Build history of the part. All positions in model axes, mm. Round coordinates to 2 decimals unless told otherwise and drop trailing zeros. Order: outer loops, then holes, each group sorted by start corner. A loop starts at its lowest first (then second) coordinate and runs counter-clockwise, first axis right, second up. Notation, with made-up numbers: (-3.5, -26) -> (54.5, -26) arc R20 ccw to (54.5, -8) -> close; hole circle Ø1 at (84, 65.5). An arc over 180 degrees is marked (long way). Answer as CSV lines item,"result". Start each with the question number.
```python
from build123d import *

# Parameters (mm, degrees)
SKETCH1_W           = 241.3
SKETCH1_H           = 114.3
SKETCH1_R           = 2.159
SKETCH1_R_2         = 3.683
SKETCH1_R_3         = 14.2875
SKETCH1_R_4         = 1.1303
SKETCH1_W_2         = 73.025
SKETCH1_H_2         = 21.59
BOSS_EXTRUDE1_DEPTH = 3.175
FILLET1_R           = 1.27
FILLET2_R           = 2.54
CUT_EXTRUDE1_START  = -1.5875
SKETCH2_R           = 1.5875
SKETCH2_W           = 75.692
SKETCH2_H           = 25.146
CUT_EXTRUDE1_DEPTH  = 1.5875


with BuildPart() as part:
    # Sketch1 → Boss-Extrude1 (new body)
    with BuildSketch(Plane(origin=(0, 0, 0), x_dir=(1, 0, 0), z_dir=(0, 1, 0))):
        Rectangle(SKETCH1_W, SKETCH1_H)
        with Locations(Location((-111.125, 47.625, 0), (0, 0, 270))):
            Circle(SKETCH1_R, mode=Mode.SUBTRACT)
        with Locations(Location((111.125, 47.625, 0), (0, 0, 90))):
            Circle(SKETCH1_R, mode=Mode.SUBTRACT)
        with Locations(Location((111.125, -47.625, 0), (0, 0, 270))):
            Circle(SKETCH1_R, mode=Mode.SUBTRACT)
        with Locations(Location((-111.125, -47.625, 0), (0, 0, 90))):
            Circle(SKETCH1_R, mode=Mode.SUBTRACT)
        with Locations(Location((-76.2, 0, 0), (0, 0, 270))):
            Circle(SKETCH1_R_2, mode=Mode.SUBTRACT)
        with Locations(Location((-31.75, 0, 0), (0, 0, 270))):
            Circle(SKETCH1_R_3, mode=Mode.SUBTRACT)
        with Locations(Location((9.5175, 19, 0), (0, 0, 270))):
            Circle(SKETCH1_R_4, mode=Mode.SUBTRACT)
        with Locations(Location((9.5175, -19, 0), (0, 0, 90))):
            Circle(SKETCH1_R_4, mode=Mode.SUBTRACT)
        with Locations(Location((92.7175, -19, 0), (0, 0, 270))):
            Circle(SKETCH1_R_4, mode=Mode.SUBTRACT)
        with Locations(Location((92.7175, 19, 0), (0, 0, 90))):
            Circle(SKETCH1_R_4, mode=Mode.SUBTRACT)
        with Locations((51.1175, 0)):
            Rectangle(SKETCH1_W_2, SKETCH1_H_2, mode=Mode.SUBTRACT)
    extrude(amount=BOSS_EXTRUDE1_DEPTH)

    # Fillet1
    fillet1_edges = [part.edges().sort_by_distance(p)[0] for p in [
        (87.63, 1.5875, 10.795),
        (87.63, 1.5875, -10.795),
        (14.605, 1.5875, -10.795),
        (14.605, 1.5875, 10.795),
    ]]
    fillet(fillet1_edges, radius=FILLET1_R)

    # Fillet2
    fillet2_edges = [part.edges().sort_by_distance(p)[0] for p in [
        (120.65, 1.5875, 57.15),
        (-120.65, 1.5875, 57.15),
        (-120.65, 1.5875, -57.15),
        (120.65, 1.5875, -57.15),
    ]]
    fillet(fillet2_edges, radius=FILLET2_R)

    # Sketch2 → Cut-Extrude1 (cut)
    # profile 1 of 21: a face of its own
    with BuildSketch(Plane(origin=(0, 0, 0), x_dir=(-1, 0, 0), z_dir=(0, -1, 0)).offset(CUT_EXTRUDE1_START)):
        with Locations((-13.2715, 12.573)):
            Circle(SKETCH2_R)
    # profile 2 of 21: a face of its own
    with BuildSketch(Plane(origin=(0, 0, 0), x_dir=(-1, 0, 0), z_dir=(0, -1, 0)).offset(CUT_EXTRUDE1_START)):
        with Locations((-88.9635, 12.573)):
            Circle(SKETCH2_R)
    # profile 3 of 21: a face of its own
    with BuildSketch(Plane(origin=(0, 0, 0), x_dir=(-1, 0, 0), z_dir=(0, -1, 0)).offset(CUT_EXTRUDE1_START)):
        with Locations((-88.9635, -12.573)):
            Circle(SKETCH2_R)
    # profile 4 of 21: a face of its own
    with BuildSketch(Plane(origin=(0, 0, 0), x_dir=(-1, 0, 0), z_dir=(0, -1, 0)).offset(CUT_EXTRUDE1_START)):
        with Locations((-13.2715, -12.573)):
            Circle(SKETCH2_R)
    # profile 5 of 21: a face of its own
    with BuildSketch(Plane(origin=(0, 0, 0), x_dir=(-1, 0, 0), z_dir=(0, -1, 0)).offset(CUT_EXTRUDE1_START)):
        with Locations((-51.1175, 0)):
            Rectangle(SKETCH2_W, SKETCH2_H)
        with BuildLine():
            ThreePointArc((-15.875, 10.795), (-14.976974388, 10.423025612), (-14.605, 9.525))
            Line((-14.605, 9.525), (-14.605, -9.525))
            ThreePointArc((-14.605, -9.525), (-14.976974388, -10.423025612), (-15.875, -10.795))
            Line((-15.875, -10.795), (-86.36, -10.795))
            ThreePointArc((-86.36, -10.795), (-87.258025612, -10.423025612), (-87.63, -9.525))
            Line((-87.63, -9.525), (-87.63, 9.525))
            ThreePointArc((-87.63, 9.525), (-87.258025612, 10.423025612), (-86.36, 10.795))
            Line((-86.36, 10.795), (-15.875, 10.795))
        make_face(mode=Mode.SUBTRACT)
    # profile 6 of 21: a face of its own
    with BuildSketch(Plane(origin=(0, 0, 0), x_dir=(-1, 0, 0), z_dir=(0, -1, 0)).offset(CUT_EXTRUDE1_START)):
        with BuildLine():
            Line((-88.9635, -10.9855), (-88.9635, -12.573))
            Line((-88.9635, -12.573), (-87.376, -12.573))
            ThreePointArc((-87.376, -12.573), (-87.840967985, -11.450467985), (-88.9635, -10.9855))
        make_face()
    # profile 7 of 21: a face of its own
    with BuildSketch(Plane(origin=(0, 0, 0), x_dir=(-1, 0, 0), z_dir=(0, -1, 0)).offset(CUT_EXTRUDE1_START)):
        with BuildLine():
            Line((-87.376, -12.573), (-88.9635, -12.573))
            Line((-88.9635, -12.573), (-88.9635, -10.9855))
            ThreePointArc((-88.9635, -10.9855), (-90.086032015, -13.695532015), (-87.376, -12.573))
        make_face()
    # profile 8 of 21: a face of its own
    with BuildSketch(Plane(origin=(0, 0, 0), x_dir=(-1, 0, 0), z_dir=(0, -1, 0)).offset(CUT_EXTRUDE1_START)):
        with BuildLine():
            Line((-88.9635, -10.9855), (-88.9635, -12.573))
            Line((-88.9635, -12.573), (-87.376, -12.573))
            ThreePointArc((-87.376, -12.573), (-87.840967985, -11.450467985), (-88.9635, -10.9855))
        make_face()
    # profile 9 of 21: a face of its own
    with BuildSketch(Plane(origin=(0, 0, 0), x_dir=(-1, 0, 0), z_dir=(0, -1, 0)).offset(CUT_EXTRUDE1_START)):
        with BuildLine():
            Line((-87.376, -12.573), (-88.9635, -12.573))
            Line((-88.9635, -12.573), (-88.9635, -10.9855))
            ThreePointArc((-88.9635, -10.9855), (-90.086032015, -13.695532015), (-87.376, -12.573))
        make_face()
    # profile 10 of 21: a face of its own
    with BuildSketch(Plane(origin=(0, 0, 0), x_dir=(-1, 0, 0), z_dir=(0, -1, 0)).offset(CUT_EXTRUDE1_START)):
        with BuildLine():
            ThreePointArc((-87.376, 12.573), (-90.086032015, 13.695532015), (-88.9635, 10.9855))
            Line((-88.9635, 10.9855), (-88.9635, 12.573))
            Line((-88.9635, 12.573), (-87.376, 12.573))
        make_face()
    # profile 11 of 21: a face of its own
    with BuildSketch(Plane(origin=(0, 0, 0), x_dir=(-1, 0, 0), z_dir=(0, -1, 0)).offset(CUT_EXTRUDE1_START)):
        with BuildLine():
            Line((-88.9635, 12.573), (-88.9635, 10.9855))
            ThreePointArc((-88.9635, 10.9855), (-87.840967985, 11.450467985), (-87.376, 12.573))
            Line((-87.376, 12.573), (-88.9635, 12.573))
        make_face()
    # profile 12 of 21: a face of its own
    with BuildSketch(Plane(origin=(0, 0, 0), x_dir=(-1, 0, 0), z_dir=(0, -1, 0)).offset(CUT_EXTRUDE1_START)):
        with BuildLine():
            ThreePointArc((-87.376, 12.573), (-90.086032015, 13.695532015), (-88.9635, 10.9855))
            Line((-88.9635, 10.9855), (-88.9635, 12.573))
            Line((-88.9635, 12.573), (-87.376, 12.573))
        make_face()
    # profile 13 of 21: a face of its own
    with BuildSketch(Plane(origin=(0, 0, 0), x_dir=(-1, 0, 0), z_dir=(0, -1, 0)).offset(CUT_EXTRUDE1_START)):
        with BuildLine():
            Line((-88.9635, 12.573), (-88.9635, 10.9855))
            ThreePointArc((-88.9635, 10.9855), (-87.840967985, 11.450467985), (-87.376, 12.573))
            Line((-87.376, 12.573), (-88.9635, 12.573))
        make_face()
    # profile 14 of 21: a face of its own
    with BuildSketch(Plane(origin=(0, 0, 0), x_dir=(-1, 0, 0), z_dir=(0, -1, 0)).offset(CUT_EXTRUDE1_START)):
        with BuildLine():
            ThreePointArc((-14.859, 12.573), (-14.394032015, 11.450467985), (-13.2715, 10.9855))
            Line((-13.2715, 10.9855), (-13.2715, 12.573))
            Line((-13.2715, 12.573), (-14.859, 12.573))
        make_face()
    # profile 15 of 21: a face of its own
    with BuildSketch(Plane(origin=(0, 0, 0), x_dir=(-1, 0, 0), z_dir=(0, -1, 0)).offset(CUT_EXTRUDE1_START)):
        with BuildLine():
            Line((-13.2715, 12.573), (-13.2715, 10.9855))
            ThreePointArc((-13.2715, 10.9855), (-12.148967985, 11.450467985), (-11.684, 12.573))
            ThreePointArc((-11.684, 12.573), (-13.2715, 14.1605), (-14.859, 12.573))
            Line((-14.859, 12.573), (-13.2715, 12.573))
        make_face()
    # profile 16 of 21: a face of its own
    with BuildSketch(Plane(origin=(0, 0, 0), x_dir=(-1, 0, 0), z_dir=(0, -1, 0)).offset(CUT_EXTRUDE1_START)):
        with BuildLine():
            ThreePointArc((-14.859, 12.573), (-14.394032015, 11.450467985), (-13.2715, 10.9855))
            Line((-13.2715, 10.9855), (-13.2715, 12.573))
            Line((-13.2715, 12.573), (-14.859, 12.573))
        make_face()
    # profile 17 of 21: a face of its own
    with BuildSketch(Plane(origin=(0, 0, 0), x_dir=(-1, 0, 0), z_dir=(0, -1, 0)).offset(CUT_EXTRUDE1_START)):
        with BuildLine():
            Line((-13.2715, 12.573), (-13.2715, 10.9855))
            ThreePointArc((-13.2715, 10.9855), (-12.148967985, 11.450467985), (-11.684, 12.573))
            ThreePointArc((-11.684, 12.573), (-13.2715, 14.1605), (-14.859, 12.573))
            Line((-14.859, 12.573), (-13.2715, 12.573))
        make_face()
    # profile 18 of 21: a face of its own
    with BuildSketch(Plane(origin=(0, 0, 0), x_dir=(-1, 0, 0), z_dir=(0, -1, 0)).offset(CUT_EXTRUDE1_START)):
        with BuildLine():
            ThreePointArc((-13.2715, -10.9855), (-14.394032015, -11.450467985), (-14.859, -12.573))
            Line((-14.859, -12.573), (-13.2715, -12.573))
            Line((-13.2715, -12.573), (-13.2715, -10.9855))
        make_face()
    # profile 19 of 21: a face of its own
    with BuildSketch(Plane(origin=(0, 0, 0), x_dir=(-1, 0, 0), z_dir=(0, -1, 0)).offset(CUT_EXTRUDE1_START)):
        with BuildLine():
            Line((-13.2715, -12.573), (-14.859, -12.573))
            ThreePointArc((-14.859, -12.573), (-13.2715, -14.1605), (-11.684, -12.573))
            ThreePointArc((-11.684, -12.573), (-12.148967985, -11.450467985), (-13.2715, -10.9855))
            Line((-13.2715, -10.9855), (-13.2715, -12.573))
        make_face()
    # profile 20 of 21: a face of its own
    with BuildSketch(Plane(origin=(0, 0, 0), x_dir=(-1, 0, 0), z_dir=(0, -1, 0)).offset(CUT_EXTRUDE1_START)):
        with BuildLine():
            ThreePointArc((-13.2715, -10.9855), (-14.394032015, -11.450467985), (-14.859, -12.573))
            Line((-14.859, -12.573), (-13.2715, -12.573))
            Line((-13.2715, -12.573), (-13.2715, -10.9855))
        make_face()
    # profile 21 of 21: a face of its own
    with BuildSketch(Plane(origin=(0, 0, 0), x_dir=(-1, 0, 0), z_dir=(0, -1, 0)).offset(CUT_EXTRUDE1_START)):
        with BuildLine():
            Line((-13.2715, -12.573), (-14.859, -12.573))
            ThreePointArc((-14.859, -12.573), (-13.2715, -14.1605), (-11.684, -12.573))
            ThreePointArc((-11.684, -12.573), (-12.148967985, -11.450467985), (-13.2715, -10.9855))
            Line((-13.2715, -10.9855), (-13.2715, -12.573))
        make_face()
    extrude(amount=CUT_EXTRUDE1_DEPTH, mode=Mode.SUBTRACT)


solid = part.part
```
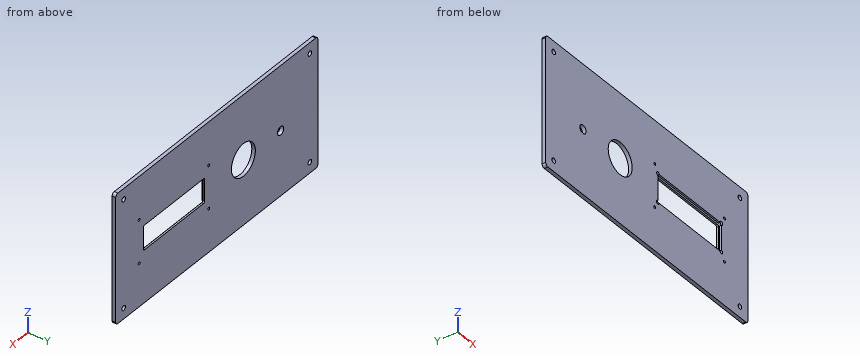
Q1. Slice it at D-D, the plane x = -76.2. Write the cut outline in (y, z) (3 decimals).
Q2. Probe L1, parallel to X at y = 1.05, z = 0; L2, parallel to X at y = 2.1, z = 48; L3, parallel to X at y = 1.7, z = 19. List the from-to ranges inside material, lowest first.
Q3. Slice it at B-B, the plane z = 0. Count the separate pieces of the cut face and the enclosed holes in it, plus the area to 3 significant figures.
Q4. Flat gauge pins, fed straight in: pin 1 Ø4 at (x, z) = (111.125, 47.625) entering from -Y; pin 2 Ø1.9 at (x, z) = (13.27, -12.57) entering from -Y. Where does each tip first touch, or does it go through?
Solutions:
1,outline,"(0, -57.15) -> (3.175, -57.15) -> (3.175, -3.683) -> (0, -3.683) -> close; (0, 3.683) -> (3.175, 3.683) -> (3.175, 57.15) -> (0, 57.15) -> close"
2,L1,"x = -120.65 to -79.88, -72.52 to -46.04, -17.46 to 13.27, 88.96 to 120.65"
2,L2,"x = -120.65 to -113.25, -109 to 109, 113.25 to 120.65"
2,L3,"x = -120.65 to 8.39, 10.65 to 91.59, 93.85 to 120.65"
3,separate pieces,"4"
3,enclosed holes,"0"
3,area,"416 mm2"
4,pin 1,"passes through"
4,pin 2,"stops at y = 1.59"
